For this review, take the finished solid that the model builds, in its own axes (mm). A direction names the side the tool comes from. Coordinates: 2 decimals unless noted, no trailing zeros. Order: outer loops, then holes, each group sorted by start corner. A loop starts at its lowest first (then second) coordinate and runs counter-clockwise, first axis right, second up. Notation, with made-up numbers: (-6, 30) -> (10, 30) arc R21 ccw to (10, 61) -> close; hole circle Ø4 at (76.5, -11). An arc over 180 degrees is marked (long way). Answer as a JSON object with one key per item and string values. Group by question number.
1) Machinability: for faces 1 (the flat face through (-3.83, -0.79, -67.25)), 2 (the flat face through (-47, -1, -65.96)), which of the approach directions +Z, -Z, +X, -X, +Y, -Y give a long, thin tool a straight path to every point of the face, cutting with its end or side? Answer none if there is none.
2) Wall thickness on L1, parallel to Z at x = -30.5, y = -0.35; L2, parallel to X at y = -0.9, z = -13.97; L3, parallel to X at y = -1, z = -66.18: over which ranges is each line inside the solid? List them lowest first.
3) Add section A-A, the plane x = -35. Write out the cut boundary in (y, z), then the cut area to 3 significant figures.
4) Draft analysis for pull direction Z (two halves, no side actions). For faces 3 (the cylindrical face through (-2.88, -0.79, -12.42)), 4 (the flat face through (-1, -1, -65.96)), 5 (the flat face through (0, -1, -33)), state which applies: +Z half, -Z half, draft (parallel to the pull), parting line (faces both ways), or undercut.
5) Add section B-B, the plane y = -0.8. Count the separate pieces of the cut face and the enclosed holes in it, then the cut area to 3 significant figures.
6) For pin 1 (0.5 mm diameter, centred on x = -1, y = -1, fed in from -Z), flat-tipped, find the tip position at first contact; note if it passes through.
from build123d import *

# Parameters (mm, degrees)
SKETCH1_R           = 1.5875
BOSS_EXTRUDE1_DEPTH = 1.6
SKETCH2_R           = 0.4
CUT_EXTRUDE1_DEPTH  = 1.65
SKETCH3_R           = 0.4
CUT_EXTRUDE2_DEPTH  = 1.65
LPATTERN1_COUNT     = 15
LPATTERN1_PITCH     = 2.54
SKETCH4_R           = 0.4
CUT_EXTRUDE3_DEPTH  = 1.65
LPATTERN2_COUNT     = 10
LPATTERN2_PITCH     = 2.54
LPATTERN3_COUNT     = 17
LPATTERN3_PITCH     = 2.54
SKETCH5_R           = 0.4
CUT_EXTRUDE4_DEPTH  = 10


with BuildPart() as part:
    # Sketch1 → Boss-Extrude1 (new body)
    with BuildSketch(Plane(origin=(0, 0, 0), x_dir=(1, 0, 0), z_dir=(0, 1, 0))):
        Polygon((0, 0), (-53.34, 0), (-53.34, 65.96), (-40.386, 65.96), (-37.846, 68.5), (-5.08, 68.5), (-2.54, 65.96), (0, 65.96), align=None)
        with Locations((-35.56, 66.04)):
            Circle(SKETCH1_R, mode=Mode.SUBTRACT)
        with Locations((-2.54, 13.97)):
            Circle(SKETCH1_R, mode=Mode.SUBTRACT)
        with Locations((-50.8, 15.24)):
            Circle(SKETCH1_R, mode=Mode.SUBTRACT)
    extrude(amount=-BOSS_EXTRUDE1_DEPTH)

    # Sketch2 → Cut-Extrude1 (cut)
    with BuildSketch(Plane(origin=(0, 0, 0), x_dir=(1, 0, 0), z_dir=(0, 1, 0))):
        with Locations((-2.54, 27.94)):
            Circle(SKETCH2_R)
    cut_extrude1 = extrude(amount=-CUT_EXTRUDE1_DEPTH, mode=Mode.SUBTRACT)

    # Sketch3 → Cut-Extrude2 (cut)
    with BuildSketch(Plane(origin=(0, 0, 0), x_dir=(1, 0, 0), z_dir=(0, 1, 0))):
        with Locations((-50.8, 18.796)):
            Circle(SKETCH3_R)
    cut_extrude2 = extrude(amount=-CUT_EXTRUDE2_DEPTH, mode=Mode.SUBTRACT)

    # LPattern1: Cut-Extrude1 ×15, 1 skipped
    with Locations(*[(0, 0, -i * LPATTERN1_PITCH) for i in range(1, LPATTERN1_COUNT) if i not in (8,)]):
        add(cut_extrude1, mode=Mode.SUBTRACT)

    # Sketch4 → Cut-Extrude3 (cut)
    with BuildSketch(Plane(origin=(0, 0, 0), x_dir=(1, 0, 0), z_dir=(0, 1, 0))):
        with Locations((-50.8, 45.72)):
            Circle(SKETCH4_R)
    cut_extrude3 = extrude(amount=-CUT_EXTRUDE3_DEPTH, mode=Mode.SUBTRACT)

    # LPattern2: Cut-Extrude2 ×10
    with Locations(*[(0, 0, -i * LPATTERN2_PITCH) for i in range(1, LPATTERN2_COUNT)]):
        add(cut_extrude2, mode=Mode.SUBTRACT)

    # LPattern3: Cut-Extrude3 ×17, 1 skipped
    with Locations(*[(0, 0, -i * LPATTERN3_PITCH) for i in range(1, LPATTERN3_COUNT) if i not in (8,)]):
        add(cut_extrude3, mode=Mode.SUBTRACT)

    # Sketch5 → Cut-Extrude4 (cut)
    with BuildSketch(Plane(origin=(0, 0, 0), x_dir=(1, 0, 0), z_dir=(0, 1, 0))):
        with Locations((-30.43, 66.18)):
            Circle(SKETCH5_R)
        with Locations((-27.89, 66.18)):
            Circle(SKETCH5_R)
        with Locations((-25.35, 66.18)):
            Circle(SKETCH5_R)
        with Locations((-25.35, 63.64)):
            Circle(SKETCH5_R)
        with Locations((-27.89, 63.64)):
            Circle(SKETCH5_R)
        with Locations((-30.43, 63.64)):
            Circle(SKETCH5_R)
    extrude(amount=-CUT_EXTRUDE4_DEPTH, mode=Mode.SUBTRACT)


solid = part.part
Output values:
{
 "1": {"face 1": "-Z, +X, +Y, -Y", "face 2": "-Z, -X, +Y, -Y"},
 "2": {"L1": "z = -68.5 to -66.57, -65.79 to -64.03, -63.25 to 0", "L2": "x = -53.34 to -51.75, -49.85 to -4.13, -0.95 to 0", "L3": "x = -40.17 to -37.14, -33.98 to -30.83, -30.03 to -28.29, -27.49 to -25.75, -24.95 to -2.76"},
 "3": {"outline": "(-1.6, -68.5) -> (0, -68.5) -> (0, -67.53) -> (-1.6, -67.53) -> close; (-1.6, -64.55) -> (0, -64.55) -> (0, 0) -> (-1.6, 0) -> close", "area": "105 mm²"},
 "4": {"face 3": "undercut", "face 4": "-Z half", "face 5": "draft"},
 "5": {"separate pieces": "1", "enclosed holes": "41", "area": "3,570 mm²"},
 "6": {"pin 1": "stops at z = -65.96"}
}
